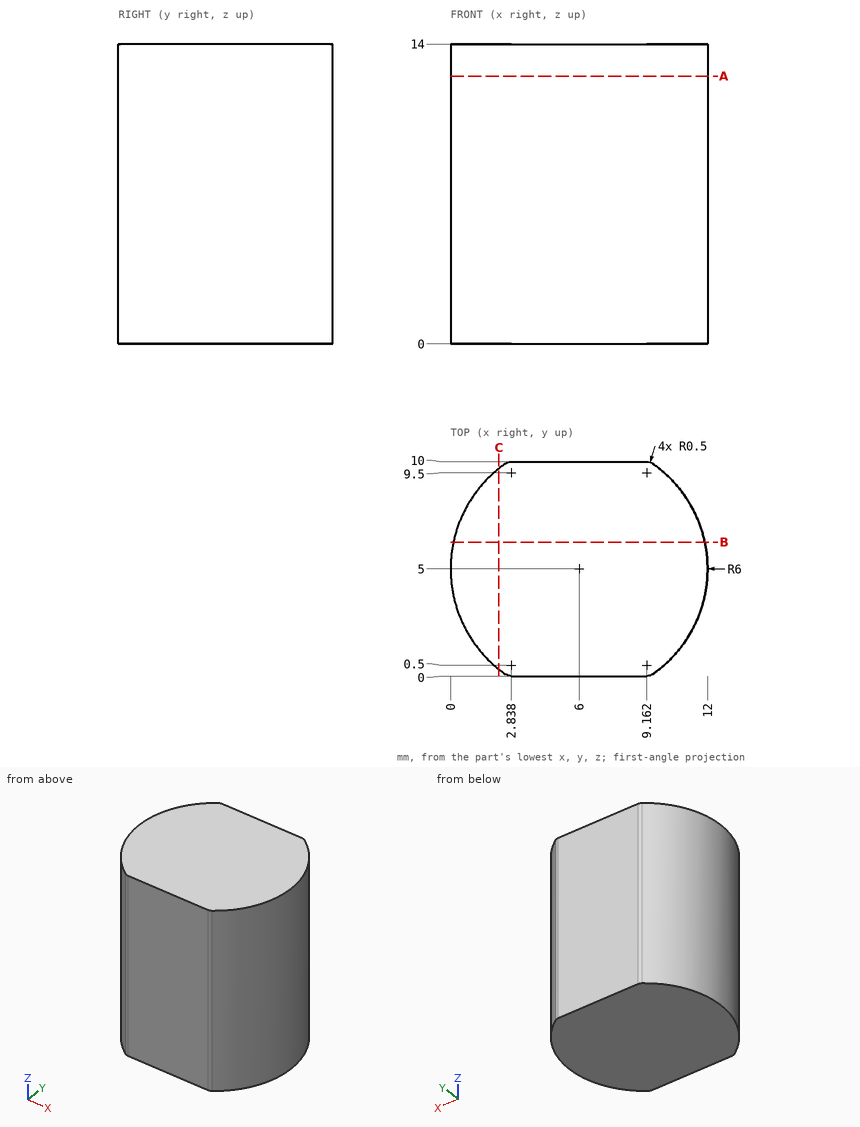
Geometry check sheet. Reference: drawing and pictorial views, mm from the part's lowest x, y, z. Coordinates: 2 decimals unless noted, no trailing zeros. Order: outer loops, then holes, each group sorted by start corner. A loop starts at its lowest first (then second) coordinate and runs counter-clockwise, first axis right, second up. Notation, with made-up numbers: M 68.5,89 L 104.5,89 A8 ccw 104.5,98 Z; hole C 41.5,65.25 d5. An arc over 180 degrees is marked long. Write each question's results on one line, items separated by ' | '. Start each with the question number.
1. Cross-section at B-B on y = 6.25. Record the cut outline in (x, z).
2. Cross-section at A-A on z = 12.5. Record the cut outline in (x, y).
3. Cross-section at C-C on x = 2.25. Record the cut outline in (y, z), and give its area (3 significant figures).
4. Material ranges on probe 1 along X at (y, z) = (0.75, 5) (1 decimal); probe 2 along X at (y, z) = (0.5, 5.5); probe 3 along Y at (x, z) = (10.25, 1) (1 decimal), recorded low to high.
Checks:
1) outline: M 0.13,0 L 11.87,0 L 11.87,14 L 0.13,14 Z
2) outline: M 2.55,0.09 A0.5 ccw 2.84,0 L 9.16,0 A0.5 ccw 9.45,0.09 A6 ccw 9.45,9.91 A0.5 ccw 9.16,10 L 2.84,10 A0.5 ccw 2.55,9.91 A6 ccw Z
3) outline: M 0.32,0 L 9.68,0 L 9.68,14 L 0.32,14 Z | area: 131 mm²
4) probe 1: x = 1.8 to 10.2 | probe 2: x = 2.03 to 9.97 | probe 3: y = 0.8 to 9.2
